Design review of the part built by this model. Coordinates are the model's own, in mm. Face numbers are marked on the shaded views. A direction names the side the tool comes from. Give positions to 0.01 mm unless a question says otherwise; leave off trailing zeros. Loops run counter-clockwise (first coordinate to the right, second up) from the corner with the lowest first, then second, coordinate; pieces in that order, holes last. Notation, with made-up numbers: (53.25, 38.25) -> (105.25, 38.25) arc R5 ccw to (105.25, 47.25) -> close; hole circle Ø2 at (-29, -17.75). An arc over 180 degrees is marked (long way). Answer in a Markdown table with one row per item. Add a question column.
(1) For line 1 (X direction, y = -1.5, z = -8); line 2 (X direction, y = -3.5, z = -9); line 3 (Z direction, x = -23, y = 0), list the stretches that pass through material, from the lowest coordinate up.
(2) Consider section D-D on z = 0.25. Write out the cut boundary in (x, y), then the cut area to 3 significant figures.
(3) Draft analysis for pull direction Y (two halves, no side actions). For the marked faces 1, 2, 3 and 4, state which applies: +Y half, -Y half, draft (parallel to the pull), parting line (faces both ways), or undercut.
(4) For the marked faces 5, 6 and 7, list the 3-axis set-ups (+Z, -Z, +X, -X, +Y, -Y) from which the entire face can be reached by the end or side of a thin tool; tool diameter is ignored.
(5) Consider section A-A on x = -14. Write out the cut boundary in (y, z).
(6) For pin 1 (2.5 mm diameter, centred on x = -11, z = -6, fed in from -Y); pin 2 (5 mm diameter, centred on y = -0.5, z = -1, fed in from +X); pin 3 (1 mm diameter, centred on y = -1, z = -10.5, fed in from -X); pin 4 (5 mm diameter, centred on x = -22.5, y = 2.5, fed in from -Z), all flat-tipped, find the tip position at first contact; note any pin that passes through.
(7) Consider section B-B on y = 0.75. Write out the cut boundary in (x, z), then the cut area to 3 significant figures.
(8) Consider section C-C on z = -3.75. Write out the cut boundary in (x, y).
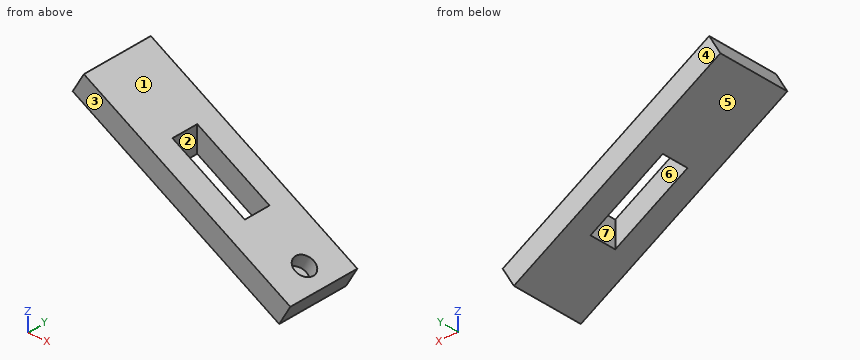
from build123d import *

# Parameters (mm, degrees)
EXTRUDE_1_DEPTH      = 5
EXTRUDE_1_DEPTH_BACK = 5
CUT_EXTRUDE_1_DEPTH  = 1.85
SKETCH_3_R           = 1.375
CUT_EXTRUDE_2_DEPTH  = 2


with BuildPart() as part:
    # Sketch 1 → Extrude 1 (new body, two sides)
    with BuildSketch(Plane(origin=(0, 0, 0), x_dir=(1, 0, 0), z_dir=(0, 1, 0))) as extrude_1_sk:
        Polygon((-24.417534462, -5.938079912), (-25.917534462, -3.340003701), (1.795278459, 12.659996299), (3.295278459, 10.061920088), align=None)
    extrude(amount=EXTRUDE_1_DEPTH)
    extrude(extrude_1_sk.sketch, amount=-EXTRUDE_1_DEPTH_BACK)

    # Sketch 2 → Cut-Extrude 1 (cut, symmetric)
    with BuildSketch(Plane(origin=(0, 0, 0), x_dir=(1, 0, 0), z_dir=(0, 1, 0))):
        Polygon((-15.35631853, 2.4), (-15.35631853, -0.706584455), (-5.65631853, 4.893713156), (-5.65631853, 8.357814772), (-15.35631853, 2.75751716), align=None)
    extrude(amount=CUT_EXTRUDE_1_DEPTH, both=True, mode=Mode.SUBTRACT)

    # Sketch 3 → Cut-Extrude 2 (cut)
    with BuildSketch(Plane(origin=(-3.533119589, 0, -6.119542637), x_dir=(0.866025404, 0, -0.5), z_dir=(0.5, 0, 0.866025404))):
        with Locations((4.884754902, 0)):
            Circle(SKETCH_3_R)
    extrude(amount=-CUT_EXTRUDE_2_DEPTH, mode=Mode.SUBTRACT)


solid = part.part
Values follow:
| question | item | result |
|---|---|---|
| 1 | line 1 | -5.66 to -0.28 |
| 1 | line 2 | -4.54 to 1.46 |
| 1 | line 3 | 1.66 to 5.12 |
| 2 | outline | (-20.57, -5) -> (-14.57, -5) -> (-14.57, -1.85) -> (-15.36, -1.85) -> (-15.36, 1.85) -> (-14.57, 1.85) -> (-14.57, 5) -> (-20.57, 5) -> close |
| 2 | area | 57.1 mm2 |
| 3 | face 1 | draft |
| 3 | face 2 | undercut |
| 3 | face 3 | -Y half |
| 3 | face 4 | +Y half |
| 4 | face 5 | -Z, -X, +Y, -Y |
| 4 | face 6 | +Z, -Z |
| 4 | face 7 | +Z, -Z, -X |
| 5 | outline | (-5, -3.54) -> (-1.85, -3.54) -> (-1.85, -0.08) -> (-5, -0.08) -> close; (1.85, -3.54) -> (5, -3.54) -> (5, -0.08) -> (1.85, -0.08) -> close |
| 6 | pin 1 | y = -5 |
| 6 | pin 2 | x = -8.76 |
| 6 | pin 3 | x = -2.81 |
| 6 | pin 4 | z = -0.08 |
| 7 | outline | (-25.92, 3.34) -> (-15.36, -2.76) -> (-15.36, 0.71) -> (-24.42, 5.94) -> close; (-5.66, -8.36) -> (1.8, -12.66) -> (3.3, -10.06) -> (1.7, -9.14) -> (0.7, -10.87) -> (-1.3, -9.72) -> (-0.3, -7.99) -> (-5.66, -4.89) -> close |
| 7 | area | 57.8 mm2 |
| 8 | outline | (-13.64, -5) -> (-7.64, -5) -> (-7.64, -1.85) -> (-13.64, -1.85) -> close; (-13.64, 1.85) -> (-7.64, 1.85) -> (-7.64, 5) -> (-13.64, 5) -> close |
